Input: part model. Units: mm. Frame: model coordinates. Face numbers are marked on the shaded views. Give positions to 0.01 mm unless a question says otherwise; leave off trailing zeros. Loops run counter-clockwise (first coordinate to the right, second up) from the corner with the lowest first, then second, coordinate; pieces in that order, holes last. Notation, with made-up numbers: (17, 59) -> (50, 59) arc R23 cw to (50, 70) -> close; hole circle Ø1 at (44, 63). An arc over 180 degrees is marked (long way). Answer as a JSON object with one key per item and string values.
```python
from build123d import *

# Parameters (mm, degrees)
SKETCH1_W           = 25.4
SKETCH1_H           = 25.4
SKETCH1_W_2         = 22.225
SKETCH1_H_2         = 22.225
BOSS_EXTRUDE1_DEPTH = 241.3
SKETCH7_R           = 1.984375
CUT_EXTRUDE8_DEPTH  = 26.4
SKETCH10_R          = 2.1828125
CUT_EXTRUDE7_DEPTH  = 25.4
SKETCH7_5_R         = 3.175
SKETCH7_5_R_2       = 1.984375
CUT_EXTRUDE9_DEPTH  = 1.5875
SKETCH13_R          = 2.5908
CUT_EXTRUDE10_DEPTH = 26.4
CUT_EXTRUDE11_REACH = 27.4
SKETCH14_R          = 7.62
SKETCH16_R          = 1.9558
CUT_EXTRUDE12_DEPTH = 26.4


with BuildPart() as part:
    # Sketch1 → Boss-Extrude1 (new body)
    with BuildSketch(Plane.XY):
        Rectangle(SKETCH1_W, SKETCH1_H)
        Rectangle(SKETCH1_W_2, SKETCH1_H_2, mode=Mode.SUBTRACT)
    extrude(amount=BOSS_EXTRUDE1_DEPTH)

    # Sketch7 → Cut-Extrude8 (cut, through all)
    with BuildSketch(Plane(origin=(0, 12.7, 0), x_dir=(1, 0, 0), z_dir=(0, 1, 0))):
        with Locations((-7.14375, -127)):
            Circle(SKETCH7_R)
        with Locations((7.14375, -127)):
            Circle(SKETCH7_R)
        with Locations((0, -76.2)):
            Circle(SKETCH7_R)
    extrude(amount=-CUT_EXTRUDE8_DEPTH, mode=Mode.SUBTRACT)

    # Sketch10 → Cut-Extrude7 (cut)
    with BuildSketch(Plane.ZY.offset(12.7)):
        with Locations((12.7, 0)):
            Circle(SKETCH10_R)
        with Locations((38.1, 0)):
            Circle(SKETCH10_R)
    extrude(amount=-CUT_EXTRUDE7_DEPTH, mode=Mode.SUBTRACT)

    # Sketch7<5> → Cut-Extrude9 (cut)
    with BuildSketch(Plane(origin=(0, 12.7, 0), x_dir=(1, 0, 0), z_dir=(0, 1, 0))):
        with Locations((-7.14375, -127)):
            Circle(SKETCH7_5_R)
        with Locations((-7.14375, -127)):
            Circle(SKETCH7_5_R_2, mode=Mode.SUBTRACT)
        with Locations((7.14375, -127)):
            Circle(SKETCH7_5_R)
        with Locations((7.14375, -127)):
            Circle(SKETCH7_5_R_2, mode=Mode.SUBTRACT)
        with Locations((0, -76.2)):
            Circle(SKETCH7_5_R)
        with Locations((0, -76.2)):
            Circle(SKETCH7_5_R_2, mode=Mode.SUBTRACT)
    extrude(amount=-CUT_EXTRUDE9_DEPTH, mode=Mode.SUBTRACT)

    # Sketch13 → Cut-Extrude10 (cut, through all)
    with BuildSketch(Plane.ZY.offset(12.7)):
        with Locations((161.29, 3.4925)):
            Circle(SKETCH13_R)
        with Locations((180.34, 3.4925)):
            Circle(SKETCH13_R)
    extrude(amount=-CUT_EXTRUDE10_DEPTH, mode=Mode.SUBTRACT)

    # Sketch14 → Cut-Extrude11 (cut, up to next)
    with BuildSketch(Plane(origin=(0, 12.7, 0), x_dir=(1, 0, 0), z_dir=(0, 1, 0)), mode=Mode.PRIVATE) as cut_extrude11_sk1:
        with Locations((0, -170.815)):
            Circle(SKETCH14_R)
    cut_extrude11_tool1 = extrude(cut_extrude11_sk1.sketch, amount=-CUT_EXTRUDE11_REACH, mode=Mode.PRIVATE) & part.part
    add(cut_extrude11_tool1.solids().sort_by_distance((0, 12.7, 170.815))[0], mode=Mode.SUBTRACT)

    # Sketch16 → Cut-Extrude12 (cut, through all)
    with BuildSketch(Plane(origin=(12.7, 0, 0), x_dir=(0, 0, -1), z_dir=(1, 0, 0))):
        with Locations((-236.474, -7.9375)):
            Circle(SKETCH16_R)
        with Locations((-236.474, 7.9375)):
            Circle(SKETCH16_R)
        with Locations((-211.074, -7.9375)):
            Circle(SKETCH16_R)
        with Locations((-211.074, 7.9375)):
            Circle(SKETCH16_R)
    extrude(amount=-CUT_EXTRUDE12_DEPTH, mode=Mode.SUBTRACT)


solid = part.part
```
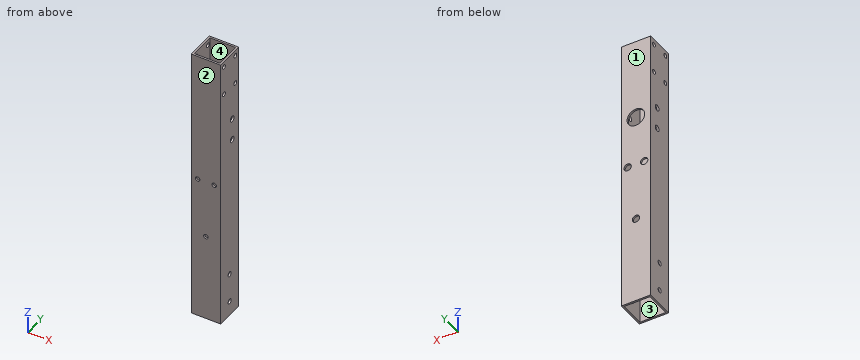
Q1. Section B-B, the plane z = 127. Return the cut outline in (x, y), then the cut area to 3 significant figures.
Evaluation:
{"outline": "(-12.7, -12.7) -> (-9.13, -12.7) -> (-9.13, -11.11) -> (-11.11, -11.11) -> (-11.11, 11.11) -> (-10.32, 11.11) -> (-10.32, 12.7) -> (-12.7, 12.7) -> close; (-5.16, -12.7) -> (5.16, -12.7) -> (5.16, -11.11) -> (-5.16, -11.11) -> close; (-3.97, 11.11) -> (3.97, 11.11) -> (3.97, 12.7) -> (-3.97, 12.7) -> close; (9.13, -12.7) -> (12.7, -12.7) -> (12.7, 12.7) -> (10.32, 12.7) -> (10.32, 11.11) -> (11.11, 11.11) -> (11.11, -11.11) -> (9.13, -11.11) -> close", "area": "118 mm2"}
Q2. Section C-C, the plane z = 22.5. Return the cut outline in (x, y), then the cut area to 3 significant figures.
Evaluation:
{"outline": "(-12.7, -12.7) -> (12.7, -12.7) -> (12.7, 12.7) -> (-12.7, 12.7) -> close; hole (-11.11, -11.11) -> (11.11, -11.11) -> (11.11, 11.11) -> (-11.11, 11.11) -> close", "area": "151 mm2"}
Q3. Draft query along Y for the marked faces 1, 2, 3 and 4. Return one class per face: +Y half, -Y half, draft (parallel to the pull), parting line (faces both ways), or undercut.
Evaluation:
{"face 1": "+Y half", "face 2": "-Y half", "face 3": "undercut", "face 4": "undercut"}
Q4. Ray query, line 1 along X through (y, z) = (-4.75, 113.5); line 2 along Y through (x, z) = (12.3, 180.34). Return the intervals inside material, ascending.
Evaluation:
{"line 1": "x = -12.7 to -11.11, 11.11 to 12.7", "line 2": "y = -12.7 to 0.9, 6.08 to 12.7"}
Q5. Section A-A, the plane z = 76.2. Return the cut outline in (x, y) (1 decimal).
Evaluation:
{"outline": "(-12.7, -12.7) -> (-2, -12.7) -> (-2, -11.1) -> (-11.1, -11.1) -> (-11.1, 11.1) -> (-3.2, 11.1) -> (-3.2, 12.7) -> (-12.7, 12.7) -> close; (2, -12.7) -> (12.7, -12.7) -> (12.7, 12.7) -> (3.2, 12.7) -> (3.2, 11.1) -> (11.1, 11.1) -> (11.1, -11.1) -> (2, -11.1) -> close"}
Q6. Pin query (flat end, axial travel): pin 1 (7 mm diameter, centred on y = 0, z = 12.7, fed in from +X); pin 2 (3.5 mm diameter, centred on x = -7.14, z = 127, fed in from -Y); pin 3 (5 mm diameter, centred on x = 0, z = 76.2, fed in from +Y). Return the tip coordinate at first contact, or that it passes through.
Evaluation:
{"pin 1": "stops at x = 12.7", "pin 2": "passes through", "pin 3": "stops at y = -11.11"}
Q7. Section D-D, the plane z = 175. Return the cut outline in (x, y).
Evaluation:
{"outline": "(-12.7, -12.7) -> (12.7, -12.7) -> (12.7, 12.7) -> (6.37, 12.7) -> (6.37, 11.11) -> (11.11, 11.11) -> (11.11, -11.11) -> (-11.11, -11.11) -> (-11.11, 11.11) -> (-6.37, 11.11) -> (-6.37, 12.7) -> (-12.7, 12.7) -> close"}
